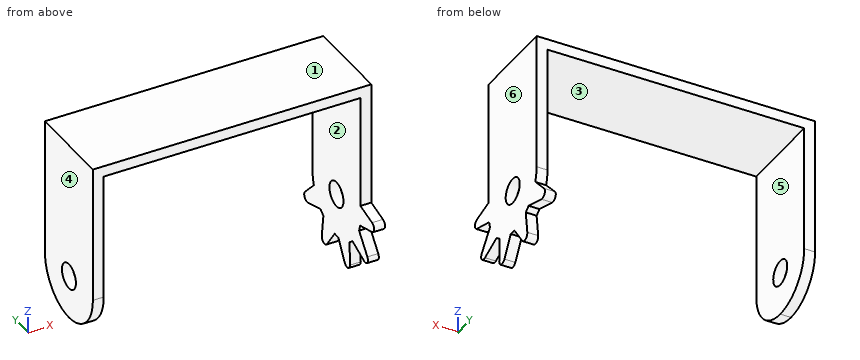
```python
from build123d import *

# Parameters (mm, degrees)
EXTRUDE_2_DEPTH     = 12
FILLET_1_R          = 6
CUT_EXTRUDE_3_REACH = 49.366
SKETCH_5_R          = 1.75
CUT_EXTRUDE_START   = -1.5
SKETCH_6_R          = 1.75
CUT_EXTRUDE_4_DEPTH = 1.5
EXTRUDE_3_DEPTH     = 1.5


with BuildPart() as part:
    # 草图2 → 凸台-拉伸2 (new body)
    with BuildSketch(Plane(origin=(0, 0, 0), x_dir=(1, 0, 0), z_dir=(0, 1, 0))):
        Polygon((0, 0), (38.4, 0), (38.4, 25), (36.9, 25), (36.9, 1.5), (1.5, 1.5), (1.5, 25), (0, 25), align=None)
    extrude(amount=EXTRUDE_2_DEPTH)

    # 圆角1
    fillet_1_edges = [part.edges().sort_by_distance(p)[0] for p in [
        (0.75, 0, -25),
        (0.75, 12, -25),
        (37.65, 0, -25),
        (37.65, 12, -25),
    ]]
    fillet(fillet_1_edges, radius=FILLET_1_R - 0.0001)  # a hair under: the kernel refuses the full size

    # 草图5 → 切除-拉伸3 (cut, up to next)
    with BuildSketch(Plane.ZY, mode=Mode.PRIVATE) as cut_extrude_3_sk1:
        with Locations((-19, 6)):
            Circle(SKETCH_5_R)
    cut_extrude_3_tool1 = extrude(cut_extrude_3_sk1.sketch, amount=-CUT_EXTRUDE_3_REACH, mode=Mode.PRIVATE) & part.part
    add(cut_extrude_3_tool1.solids().sort_by_distance((0, 6, -19))[0], mode=Mode.SUBTRACT)

    # 草图6 → 切除-拉伸4 (cut)
    with BuildSketch(Plane(origin=(38.4, 0, 0), x_dir=(0, 0, -1), z_dir=(1, 0, 0)).offset(CUT_EXTRUDE_START)):
        with Locations(Location((19, 6, 0), (0, 0, 180))):
            Circle(SKETCH_6_R)
    extrude(amount=CUT_EXTRUDE_4_DEPTH, mode=Mode.SUBTRACT)

    # 草图7 → 凸台-拉伸3 (add)
    with BuildSketch(Plane(origin=(38.4, 0, 0), x_dir=(0, 0, -1), z_dir=(1, 0, 0))):
        with BuildLine():
            Line((20.999709003, 11.656957124), (23.241440486, 13.870627343))
            ThreePointArc((23.241440486, 13.870627343), (24.09053112, 13.974522864), (24.406127138, 13.179445297))
            Line((24.406127138, 13.179445297), (23.488407969, 9.981732526))
            ThreePointArc((23.488407969, 9.981732526), (22.350449197, 10.977397932), (20.999709003, 11.656957124))
        make_face()
        with BuildLine():
            Line((27.659538401, 8.404795226), (24.984818637, 6.42655115))
            ThreePointArc((24.984818637, 6.42655115), (24.68813794, 7.909211035), (24.03021312, 9.27062012))
            Line((24.03021312, 9.27062012), (27.156295325, 9.662163121))
            ThreePointArc((27.156295325, 9.662163121), (27.893171802, 9.227695353), (27.659538401, 8.404795226))
        make_face()
        with BuildLine():
            Line((27.334020294, 2.636259354), (24.007743744, 2.695079034))
            ThreePointArc((24.007743744, 2.695079034), (24.674957273, 4.051959971), (24.981763759, 5.53255767))
            Line((24.981763759, 5.53255767), (27.700207796, 3.940151347))
            ThreePointArc((27.700207796, 3.940151347), (28.02032399, 3.146882915), (27.334020294, 2.636259354))
        make_face()
        with BuildLine():
            Line((23.564107276, -1.742064981), (20.961001817, 0.329508674))
            ThreePointArc((20.961001817, 0.329508674), (22.316354676, 0.999820837), (23.461091399, 1.987686013))
            Line((23.461091399, 1.987686013), (24.648382507, -0.93053874))
            ThreePointArc((24.648382507, -0.93053874), (24.419436534, -1.754755292), (23.564107276, -1.742064981))
        make_face()
        with BuildLine():
            Line((17.907879211, -2.920645581), (17.103790939, 0.307514497))
            ThreePointArc((17.103790939, 0.307514497), (18.587124847, 0.014222347), (20.096679766, 0.101076921))
            Line((20.096679766, 0.101076921), (19.262118462, -2.936883465))
            ThreePointArc((19.262118462, -2.936883465), (18.578732164, -3.451404943), (17.907879211, -2.920645581))
        make_face()
    extrude(amount=-EXTRUDE_3_DEPTH)


solid = part.part
```
Source: CAD feature listing. Evaluate the final solid. Frame: model axes, mm. Face numbers are marked on the shaded views. A direction names the side the tool comes from. Give positions to 0.01 mm unless a question says otherwise; leave off trailing zeros. Order: outer loops, then holes, each group sorted by start corner. A loop starts at its lowest first (then second) coordinate and runs counter-clockwise, first axis right, second up.
(1) Contact query for flat-ended pins moving along their axis: P1, Ø3, axis at y = 6, z = -19, coming from the +X side; P2, Ø1.5, axis at x = 21.5, y = 8.5, coming from the -Z side; P3, Ø8, axis at x = 25, z = -3.5, coming from the -Y side. Output: stop coordinate, or through.
(2) Section query D-D (z = -22.25). Return the cut outline in (x, y).
(3) Section query A-A (z = -16.75). Return the cut outline in (x, y), plus the area to 3 significant figures.
(4) Section query C-C (x = 5). Return the cut outline in (y, z).
(5) Material intervals for line 1 along X through (y, z) = (10.75, -16.5); line 2 along Z through (x, y) = (37.6, 6); line 3 along Y through (x, z) = (0.4, -19), sorted ascending.
(6) Pull-direction query (X, two-part tool) for the marked faces 1, 2, 3 and 4; classes: +X half, -X half, draft (parallel to the pull), parting line (faces both ways), or undercut.
(7) Section query B-B (y = 10.5). Return the cut outline in (x, z), plus the area to 3 significant figures.
(8) Access query for the marked faces 5 and 6. Directions: +Z, -Z, +X, -X, +Y, -Y. A direction counts if a zero-diameter tool reaches every point of the face in a straight line with its end or side. Return the directions, or none.
Outcome:
1. P1: passes through
1. P2: stops at z = -1.5
1. P3: stops at y = 0
2. outline: (0, 0.96) - (1.5, 0.96) - (1.5, 11.04) - (0, 11.04) - close; (36.9, -0.7) - (38.4, -0.7) - (38.4, 12.89) - (36.9, 12.89) - close
3. outline: (0, 0) - (1.5, 0) - (1.5, 12) - (0, 12) - close; (36.9, 0) - (38.4, 0) - (38.4, 12) - (36.9, 12) - close
3. area: 36.0 mm2
4. outline: (0, -1.5) - (12, -1.5) - (12, 0) - (0, 0) - close
5. line 1: x = 0 to 1.5, 36.9 to 38.4
5. line 2: z = -25 to -20.75, -17.25 to 0
5. line 3: y = 0 to 4.25, 7.75 to 12
6. face 1: draft
6. face 2: undercut
6. face 3: undercut
6. face 4: -X half
7. outline: (0, -22.97) - (1.5, -22.97) - (1.5, -1.5) - (36.9, -1.5) - (36.9, -23.64) - (38.4, -23.64) - (38.4, 0) - (0, 0) - close
7. area: 123 mm2
8. face 5: -Z, +Y, -Y
8. face 6: +Z, -Z, +X, +Y, -Y
